Input: dimensioned drawing with shaded views. Units: mm. Origin: part minimum x, y, z. Coordinates: 2 decimals unless noted, no trailing zeros. Order: outer loops, then holes, each group sorted by start corner. A loop starts at its lowest first (then second) coordinate and runs counter-clockwise, first axis right, second up. Notation, with made-up numbers: M 57.25,-40 L 99.25,-40 A16 cw 99.25,-25 Z; hole C -30.75,4 d1. An arc over 180 degrees is marked long. Use CSV: the item, a comma, the result in double quotes. Start each with the question number.
1. First-contact query: P1, Ø4, axis at y = 51, z = 4.76, coming from the -X side; P2, Ø3.5, axis at y = 51, z = 4.76, coming from the +X side. Flat tips, straight axial feed; report the tip coordinate or a pass-through.
2. Section query A-A on x = 80.8. State how many separate pieces and enclosed holes the cut face has, and give its area (3 significant figures).
3. Section query B-B on y = 43.75. Return the cut outline in (x, z) (1 decimal), and give its area (3 significant figures).
4. Section query D-D on y = 86. Return the cut outline in (x, z) (1 decimal).
5. Material intervals for line 1 (Y direction, x = 80.8, z = 7.75); line 2 (X direction, y = 128.25, z = 5); line 3 (Y direction, x = 19, z = 3.75) (1 decimal), sorted ascending.
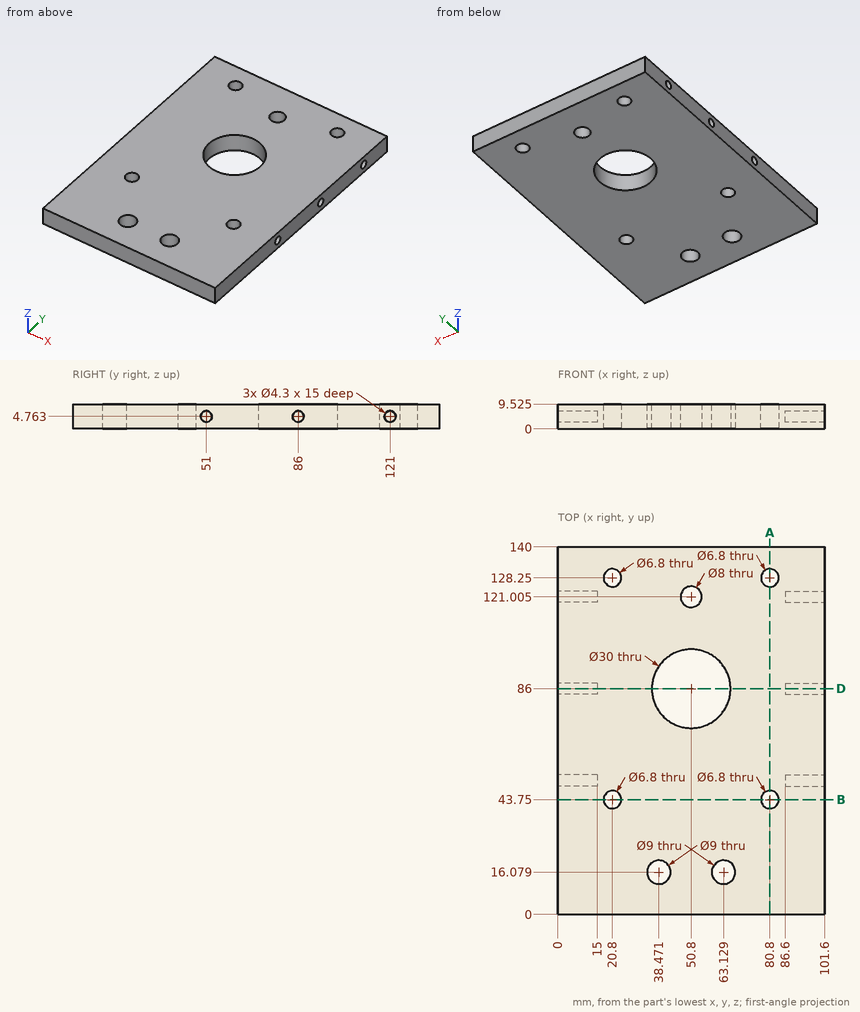
Results list:
1,P1,"stops at x = 15"
1,P2,"stops at x = 86.6"
2,separate pieces,"3"
2,enclosed holes,"0"
2,area,"1,200 mm²"
3,outline,"M 0,0 L 17.4,0 L 17.4,9.5 L 0,9.5 Z; M 24.2,0 L 77.4,0 L 77.4,9.5 L 24.2,9.5 Z; M 84.2,0 L 101.6,0 L 101.6,9.5 L 84.2,9.5 Z"
3,area,"838 mm²"
4,outline,"M 0,0 L 35.8,0 L 35.8,9.5 L 0,9.5 L 0,6.9 L 15,6.9 L 15,2.6 L 0,2.6 Z; M 65.8,0 L 101.6,0 L 101.6,2.6 L 86.6,2.6 L 86.6,6.9 L 101.6,6.9 L 101.6,9.5 L 65.8,9.5 Z"
5,line 1,"y = 0 to 40.35, 47.15 to 124.85, 131.65 to 140"
5,line 2,"x = 0 to 17.4, 24.2 to 77.4, 84.2 to 101.6"
5,line 3,"y = 0 to 40.9, 46.6 to 125.4, 131.1 to 140"
